Check sheet for the modelled part. Datum: model origin and axes. Units: mm. A direction names the side the tool comes from. Give positions to 0.01 mm unless a question says otherwise; leave off trailing zeros. Write each loop counter-clockwise with the first axis right and the second up, starting at its lowest first coordinate (ties: lowest second). Pieces come first, ordered by that corner, then holes. Notation, with made-up numbers: (52, 37.5) -> (67, 37.5) arc R22 ccw to (67, 58.5) -> close; hole circle Ø10 at (75, 83). An arc over 180 degrees is marked (long way). Return JSON: item names as keys, results as strings.
Autodesk Inventor part; units mm, degrees
ref_plane "YZ Plane" through (0, 0, 0) normal (1, 0, 0) x (0, 1, 0)
ref_plane "XZ Plane" through (0, 0, 0) normal (0, 1, 0) x (-1, 0, 0)
ref_plane "XY Plane" through (0, 0, 0) normal (0, 0, 1) x (1, 0, 0)
sketch "Sketch1" plane through (0, 0, 0) normal (0, 0, 1) x (1, 0, 0)
  line L0 (98, 0) -> (98, -90)
  line L1 (98, -90) -> (-90, -90)
  line L2 (-90, -90) -> (-90, 0)
  line L3 (126, 4) -> (126, 0)
  line L4 (126, 0) -> (-118, 0)
  line L5 (-118, 0) -> (-118, 4)
  line L6 (-86, 4) -> (94, 4)
  line L7 (94, 4) -> (94, -86)
  line L8 (94, -86) -> (-86, -86)
  line L9 (-86, -86) -> (-86, 4)
  line L10 (-90, 0) -> (-86, 0)
  line L11 (94, 0) -> (98, 0)
  line L12 (-118, 4) -> (-86, 4)
  line L13 (94, 4) -> (126, 4)
  point P0 (0, 0)
  point P1 (6, -4)
  point P2 (126, 2)
  point P3 (98, 0)
  point P4 (-118, 2)
  dimension "d0" = 188
  dimension "d1" = 90
  dimension "d3" = 90
  dimension "d4" = 244
  dimension "d5" = 120
  dimension "d8" = 90
  dimension "d9" = 180
  dimension "d10" = 4
  dimension "d13" = 0
  dimension "d14" = 4
  dimension "d72" = 32
extrude "Extrusion1" add sketch "Sketch1" along normal blind 90 contours L4 L7 L13 L3 | L0 L1 L2 L4 L9 L8 L7 | L4 L5 L12 L9
fillet "Fillet1" radius 2 4 edges at (-86, -86, 45) (-86, 4, 45) (94, 4, 45) (98, -90, 45)
fillet "Fillet2" radius 2 2 edges at (-90, -90, 45) (94, -86, 45)
sketch "Sketch7" plane through (-118, 0, 0) normal (0, -1, 0) x (1, 0, 0)
  line L0 (0, 0) -> (0, 90)
  line L1 (0, 0) -> (28, 0)
  line L2 (244, 0) -> (244, 90)
  line L3 (216, 0) -> (244, 0)
  point P0 (118, 0)
  point P1 (16, 20)
  point P2 (16, 60)
  point P3 (228, 20)
  point P4 (228, 60)
  dimension "d73" = 16
  dimension "d74" = 16
  dimension "d75" = 20
  dimension "d76" = 40
  dimension "d77" = 16
  dimension "d78" = 16
  dimension "d79" = 20
  dimension "d80" = 40
hole "Hole6" at (-102, 0, 20) at (-102, 0, 60) at (110, 0, 20) at (110, 0, 60) direction (0, 1, 0) diameter 4.917 end through all
equation "\"d86\" = Thickness"
equation "\"BendRadius\" = Thickness"
equation "\"BendReliefWidth\" = Thickness"
equation "\"BendReliefDepth\" = 0.5 * Thickness"
equation "\"CornerReliefSize\" = 4 * Thickness"
equation "\"MinimumRemnant\" = 2 * Thickness"
equation "\"TransitionRadius\" = BendRadius"
equation "\"JacobiRadiusSize\" = BendRadius"
equation "\"GapSize\" = Thickness"
properties part number "Top joint housing"
(1) Thickness scan on L1, parallel to X at y = 1.25, z = 60; L2, parallel to Z at x = -102, y = 1.85; L3, parallel to X at y = -33, z = 51.5. Record the ranges inside material, lowest first.
Reply:
{"L1": "-118 to -104.46, -99.54 to -86, 94 to 107.54, 112.46 to 126", "L2": "0 to 17.54, 22.46 to 57.54, 62.46 to 90", "L3": "-90 to -86, 94 to 98"}
(2) Set-up check for faces 1 (the flat face through (98, -43, 44)), 2 (the flat face through (-86, -42, 44)), 3 (the flat face through (-104, 0, 44)), 4 (the cylindrical face through (112.2, 2, 58.9)): record each of +Z, -Z, +X, -X, +Y, -Y from which the full face is reachable in a straight line by a thin tool's end or side.
Reply:
{"face 1": "+Z, -Z, +X, -Y", "face 2": "+Z, -Z, +Y", "face 3": "+Z, -Z, -X, -Y", "face 4": "+Y, -Y"}
(3) Depth check by flat-ended pin: pin 1 Ø2 at (y, z) = (-78.5, 49) entering from +X; pin 2 Ø8 at (y, z) = (-74.5, 49.5) entering from -X; pin 3 Ø8 at (x, z) = (110, 20) entering from -Y. Enter the tip coordinate at first touch or a pass-through.
Reply:
{"pin 1": "x = 98", "pin 2": "x = -90", "pin 3": "y = 0"}
(4) Cross-section at D-D on z = 65.5. Enter the section's corners in (x, y), then the cut area to 3 significant figures.
Reply:
{"outline": "(-118, 0) -> (-90, 0) -> (-90, -88) arc R2 ccw to (-88, -90) -> (96, -90) arc R2 ccw to (98, -88) -> (98, 0) -> (126, 0) -> (126, 4) -> (96, 4) arc R2 ccw to (94, 2) -> (94, -84) arc R2 cw to (92, -86) -> (-84, -86) arc R2 cw to (-86, -84) -> (-86, 2) arc R2 ccw to (-88, 4) -> (-118, 4) -> close", "area": "1,690 mm^2"}
(5) Release check for a two-part mould opening along X. For faces 5 (the flat face through (111, 4, 44)), 6 (the flat face through (5, -86, 44)), 7 (the flat face through (-90, -45, 44)) record: pulls with the +X half, pulls with the -X half, needs draft (parallel to the pull), parting line crosses it, or undercut.
Reply:
{"face 5": "needs draft", "face 6": "undercut", "face 7": "pulls with the -X half"}
(6) Cross-section at A-A on y = -76.5. Enter the section's corners in (x, z), then the cut area to 3 significant figures.
Reply:
{"outline": "(-90, 0) -> (-86, 0) -> (-86, 90) -> (-90, 90) -> close; (94, 0) -> (98, 0) -> (98, 90) -> (94, 90) -> close", "area": "720 mm^2"}
(7) Cross-section at C-C on x = 110. Enter the section's corners in (y, z), then the cut area to 3 significant figures.
Reply:
{"outline": "(0, 0) -> (4, 0) -> (4, 17.54) -> (0, 17.54) -> close; (0, 22.46) -> (4, 22.46) -> (4, 57.54) -> (0, 57.54) -> close; (0, 62.46) -> (4, 62.46) -> (4, 90) -> (0, 90) -> close", "area": "321 mm^2"}
(8) Cross-section at B-B on z = 20. Enter the section's corners in (x, y), then the cut area to 3 significant figures.
Reply:
{"outline": "(-118, 0) -> (-104.46, 0) -> (-104.46, 4) -> (-118, 4) -> close; (-99.54, 0) -> (-90, 0) -> (-90, -88) arc R2 ccw to (-88, -90) -> (96, -90) arc R2 ccw to (98, -88) -> (98, 0) -> (107.54, 0) -> (107.54, 4) -> (96, 4) arc R2 ccw to (94, 2) -> (94, -84) arc R2 cw to (92, -86) -> (-84, -86) arc R2 cw to (-86, -84) -> (-86, 2) arc R2 ccw to (-88, 4) -> (-99.54, 4) -> close; (112.46, 0) -> (126, 0) -> (126, 4) -> (112.46, 4) -> close", "area": "1,650 mm^2"}
